Geometry: final body of the model. Coordinates: model frame, mm. A direction names the side the tool comes from. Give positions to 0.01 mm unless a question says otherwise; leave off trailing zeros. Write each loop counter-clockwise with the first axis right and the second up, starting at its lowest first coordinate (ties: lowest second). Pieces come first, ordered by that corner, then holes. Notation, with made-up numbers: (40, 46.5) - (55, 46.5) arc R14 cw to (55, 72.5) - close; hole circle Ø6 at (-10.75, 2.25). An arc over 180 degrees is marked (long way). One line per question, with ' | ' between items. Start each with the question number.
```python
from build123d import *

# Parameters (mm, degrees)
RAIL_PROFILE_W     = 6.35
RAIL_PROFILE_H     = 6.35
BACKCLIP_DEPTH     = 12.7
FRONTCLIP_DEPTH    = 12.7
SKETCH8_R          = 2.667
CUT_EXTRUDE1_DEPTH = 179.88374375
FILLET1_R          = 2.54
CUT_EXTRUDE3_DEPTH = 181.090926708
FILLET3_R          = 6.35
FILLET5_R          = 1.27
FILLET10_R         = 6.35


with BuildPart() as part:
    # Sweep1: sweep along a path in rail_path
    with BuildLine(Plane(origin=(0, 0, 0), x_dir=(1, 0, 0), z_dir=(0, 1, 0))) as sweep1_path:
        Line((31.75, 165.1), (28.575, 123.825))
        Line((28.575, 123.825), (28.575, 111.125))
        Line((28.575, 111.125), (28.575, -111.125))
        Line((28.575, -111.125), (-28.575, -111.125))
        Line((-28.575, -111.125), (-28.575, 111.125))
        Line((-28.575, 111.125), (-28.575, 123.825))
        Line((-28.575, 123.825), (-31.75, 165.1))
    # rail_profile → Sweep1 (sweep)
    with BuildSketch(Plane.XY):
        with Locations((31.75, 3.175)):
            Rectangle(RAIL_PROFILE_W, RAIL_PROFILE_H)
    sweep(path=sweep1_path.line, transition=Transition.RIGHT)

    # BackClipProfile → BackClip (add, symmetric)
    with BuildSketch(Plane(origin=(0, 0, 70.485), x_dir=(-1, 0, 0), z_dir=(0, 0, -1))):
        Polygon((-34.925, -8.89), (-34.925, 0), (-28.575, 0), (-28.575, -8.89), (-31.75, -8.89), (-31.75, -17.272), (-34.925, -17.272), align=None)
    backclip = extrude(amount=BACKCLIP_DEPTH, both=True)

    # BackClipMirror: BackClip across plane
    add(backclip.mirror(Plane(origin=(0, 0, 0), x_dir=(0, 0, 1), z_dir=(1, 0, 0))))

    # FrontClipProfile → FrontClip (add, symmetric)
    with BuildSketch(Plane(origin=(0, 0, -111.125), x_dir=(-1, 0, 0), z_dir=(0, 0, -1))):
        Polygon((-31.75, -17.272), (-31.75, -8.89), (-28.575, -8.89), (-28.575, 0), (-34.925, 0), (-34.925, -8.89), (-34.925, -17.272), align=None)
    frontclip = extrude(amount=FRONTCLIP_DEPTH, both=True)

    # FrontClipMirror: FrontClip across plane
    add(frontclip.mirror(Plane(origin=(0, 0, 0), x_dir=(0, 0, 1), z_dir=(1, 0, 0))))

    # Sketch8 → Cut-Extrude1 (cut, symmetric)
    with BuildSketch(Plane.ZY.offset(-28.575)):
        with Locations((70.485, 0)):
            Circle(SKETCH8_R)
    cut_extrude1 = extrude(amount=CUT_EXTRUDE1_DEPTH, both=True, mode=Mode.SUBTRACT)

    # Fillet1
    fillet1_edges = [part.edges().sort_by_distance(p)[0] for p in [
        (33.3375, -17.272, -98.425),
        (33.3375, -17.272, -123.825),
        (-33.3375, -17.272, -123.825),
        (-33.3375, -17.272, -98.425),
        (33.3375, -17.272, 83.185),
        (33.3375, -17.272, 57.785),
        (-33.3375, -17.272, 57.785),
        (-33.3375, -17.272, 83.185),
    ]]
    fillet(fillet1_edges, radius=FILLET1_R)

    # Mirror2: Cut-Extrude1 across plane
    add(cut_extrude1.mirror(Plane(origin=(0, 0, -20.32), x_dir=(1, 0, 0), z_dir=(0, 0, -1))), mode=Mode.SUBTRACT)

    # Sketch10 → Cut-Extrude3 (cut, symmetric)
    with BuildSketch(Plane.ZY.offset(-31.75)):
        with BuildLine():
            Line((64.135, -9.906), (76.835, -9.906))
            ThreePointArc((76.835, -9.906), (78.994, -12.065), (76.835, -14.224))
            Line((76.835, -14.224), (64.135, -14.224))
            ThreePointArc((64.135, -14.224), (61.976, -12.065), (64.135, -9.906))
        make_face()
    cut_extrude3 = extrude(amount=CUT_EXTRUDE3_DEPTH, both=True, mode=Mode.SUBTRACT)

    # Mirror3: Cut-Extrude3 across plane
    add(cut_extrude3.mirror(Plane(origin=(0, 0, -20.32), x_dir=(1, 0, 0), z_dir=(0, 0, -1))), mode=Mode.SUBTRACT)

    # Fillet3
    fillet3_edges = [part.edges().sort_by_distance(p)[0] for p in [
        (31.75, 3.175, -165.1),
        (-31.75, 3.175, -165.1),
    ]]
    fillet(fillet3_edges, radius=FILLET3_R - 0.0001)  # a hair under: the kernel refuses the full size

    # Fillet5
    fillet5_edges = [part.edges().sort_by_distance(p)[0] for p in [
        (-38.081295983, 3.175, -164.612977232),
        (38.081295983, 3.175, -164.612977232),
    ]]
    fillet(fillet5_edges, radius=FILLET5_R)

    # Fillet10
    fillet10_edges = [part.edges().sort_by_distance(p)[0] for p in [
        (31.75, 0, -98.425),
        (31.75, 0, -123.825),
        (-31.75, 0, -123.825),
        (-31.75, 0, -98.425),
        (31.75, 0, 83.185),
        (31.75, 0, 57.785),
        (-31.75, 0, 57.785),
        (-31.75, 0, 83.185),
    ]]
    fillet(fillet10_edges, radius=FILLET10_R)


solid = part.part
```
1) Reachability of faces 4 (the cylindrical face through (-31.79, 0.12, 67.82)), 5 (the flat face through (-33, -10, -98.425)), 6 (the flat face through (28.575, 2, -8)), 7 (the flat face through (31.75, -15, 70)), 8 (the cylindrical face through (31.794, -1.811, -125.735)) from +Z, -Z, +X, -X, +Y, -Y: full face, straight path, thin tool, end or side. Return the list, or none.
2) First-contact query: pin 1 Ø6 at (x, y) = (13, 3.5) entering from -Z (3 decimals); pin 2 Ø6.5 at (y, z) = (-15, 70) entering from +X (3 decimals); pin 3 Ø4 at (y, z) = (-1, -134) entering from -X. Flat tips, straight axial feed; report the tip coordinate or a pass-through.
3) Line query: L1, parallel to Z at x = 32.5, y = -7.75 (3 decimals); L2, parallel to X at y = -16.5, z = 82 (3 decimals); L3, parallel to Y at x = -29, z = 38.5. Output: solid intervals per line, ascending.
4) Pull-direction query (X, two-part tool) for faces 1 (the flat face through (29.9, 2.91, -141.05)), 2 (the flat face through (32, -10, 83.185)), 3 (the flat face through (34.925, 4, -16)); classes: +X half, -X half, draft (parallel to the pull), parting line (faces both ways), or undercut.
5) Section B-B, the plane x = -20.5. Output: boundary loops of the cut face in (y, z) (3 decimals), plus the area to 3 significant figures.
6) Section A-A, the plane z = 11.5. Output: boundary loops of the cut face in (x, y) (3 decimals), plus the area to 3 significant figures.
Answer key:
1) face 4: +X, -X | face 5: +X, -X, -Y | face 6: -Z, +Y, -Y | face 7: +Z, -Z, -Y | face 8: -Z, +X, -X, -Y
2) pin 1: z = 111.125 | pin 2: x = 34.925 | pin 3: x = -35.86
3) L1: -123.825 to -98.425, 57.785 to 83.185 | L2: -34.925 to -31.75, 31.75 to 34.925 | L3: 0 to 6.35
4) face 1: undercut | face 2: draft | face 3: +X half
5) outline: (0, 111.125) - (6.35, 111.125) - (6.35, 117.475) - (0, 117.475) - close | area: 40.3 mm^2
6) outline: (-34.925, 0) - (-28.575, 0) - (-28.575, 6.35) - (-34.925, 6.35) - close; (28.575, 0) - (34.925, 0) - (34.925, 6.35) - (28.575, 6.35) - close | area: 80.6 mm^2
